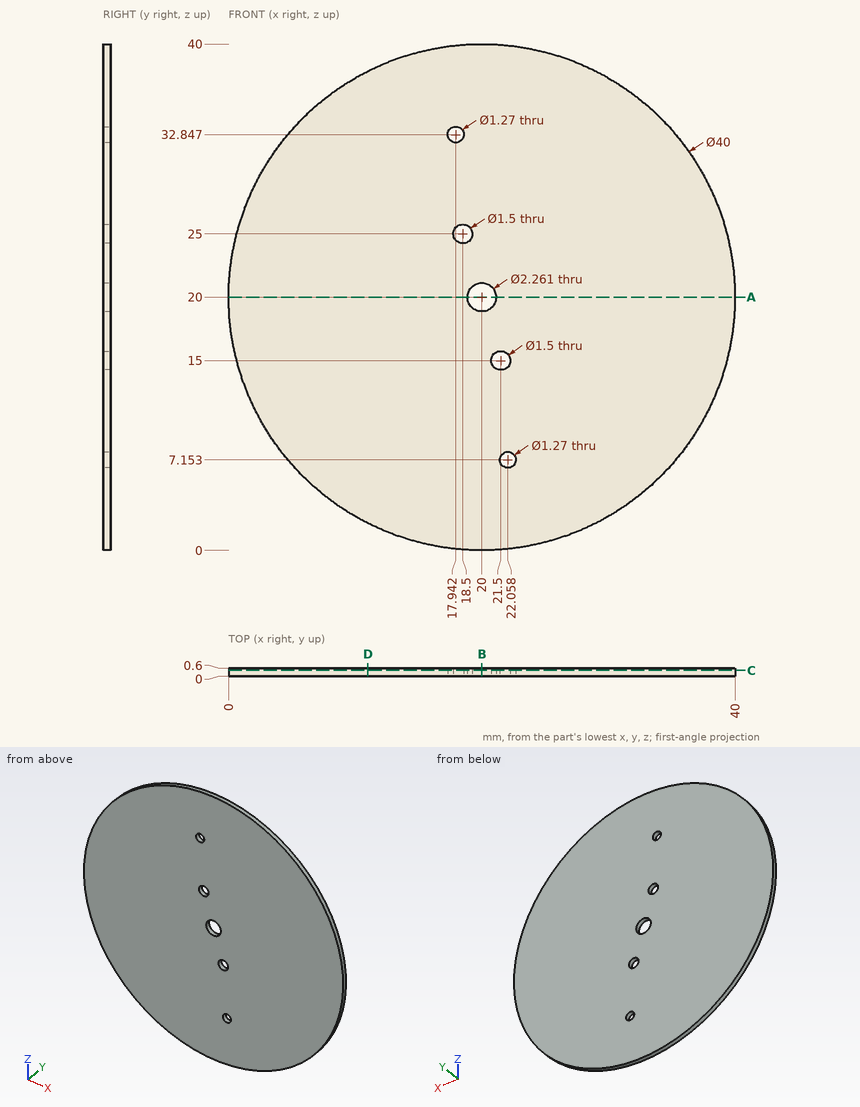
Geometry: see drawing. Coordinates: mm, zero at the bounding-box minimum. Give positions to 0.01 mm unless a question says otherwise; leave off trailing zeros. Order: outer loops, then holes, each group sorted by start corner. A loop starts at its lowest first (then second) coordinate and runs counter-clockwise, first axis right, second up.
1. Cut plane A-A (z = 20). Return loops of the section in (x, y).
Computed:
outline: (0, 0) - (18.87, 0) - (18.87, 0.6) - (0, 0.6) - close; (21.13, 0) - (40, 0) - (40, 0.6) - (21.13, 0.6) - close
2. Line query: probe 1 along Z at (x, y) = (24, 0.4) (1 decimal); probe 2 along X at (y, z) = (0.1, 11.5) (1 decimal). Output: solid intervals per line, ascending.
Computed:
probe 1: z = 0.4 to 39.6
probe 2: x = 1.9 to 38.1
3. Cut plane B-B (x = 20). Return loops of the section in (y, z).
Computed:
outline: (0, 0) - (0.6, 0) - (0.6, 18.87) - (0, 18.87) - close; (0, 21.13) - (0.6, 21.13) - (0.6, 40) - (0, 40) - close
4. Cut plane D-D (x = 11). Return loops of the section in (y, z).
Computed:
outline: (0, 2.14) - (0.6, 2.14) - (0.6, 37.86) - (0, 37.86) - close
5. Cut plane C-C (y = 0.45). State how many separate pieces and enclosed holes the cut face has, and give its area (3 significant figures).
Computed:
separate pieces: 1
enclosed holes: 5
area: 1,250 mm2
6. Pin query (flat end, axial travel): pin 1 Ø1.5 at (x, z) = (12, 14) entering from -Y. Return the tip coordinate at first contact, or that it passes through.
Computed:
pin 1: stops at y = 0
